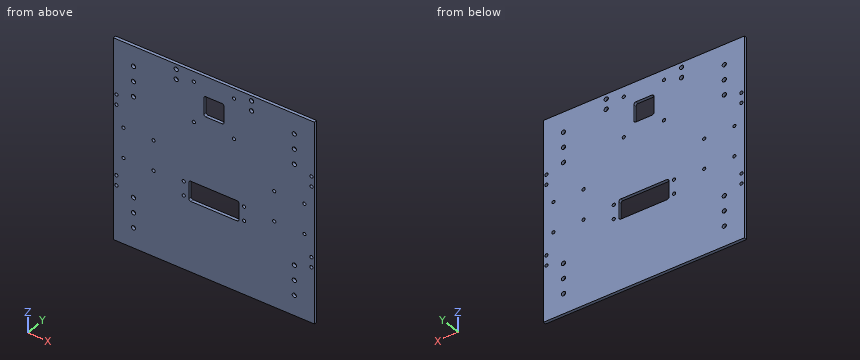
from build123d import *

# Parameters (mm, degrees)
SKETCH_1_W      = 200
SKETCH_1_H      = 200
SKETCH_1_R      = 1.6
SKETCH_1_R_2    = 2.1
EXTRUDE_1_DEPTH = 3


with BuildPart() as part:
    # 草图1 → 凸台-拉伸1 (new body)
    with BuildSketch(Plane(origin=(0, 0, 0), x_dir=(1, 0, 0), z_dir=(0, 1, 0))):
        Rectangle(SKETCH_1_W, SKETCH_1_H)
        with Locations(Location((-97, 35, 0), (0, 0, 270))):
            Circle(SKETCH_1_R, mode=Mode.SUBTRACT)
        with Locations(Location((-97, 45, 0), (0, 0, 270))):
            Circle(SKETCH_1_R, mode=Mode.SUBTRACT)
        with Locations(Location((-97, -45, 0), (0, 0, 90))):
            Circle(SKETCH_1_R, mode=Mode.SUBTRACT)
        with Locations(Location((-97, -35, 0), (0, 0, 90))):
            Circle(SKETCH_1_R, mode=Mode.SUBTRACT)
        with Locations(Location((97, -45, 0), (0, 0, 270))):
            Circle(SKETCH_1_R, mode=Mode.SUBTRACT)
        with Locations(Location((97, -35, 0), (0, 0, 270))):
            Circle(SKETCH_1_R, mode=Mode.SUBTRACT)
        with Locations(Location((97, 35, 0), (0, 0, 90))):
            Circle(SKETCH_1_R, mode=Mode.SUBTRACT)
        with Locations(Location((97, 45, 0), (0, 0, 90))):
            Circle(SKETCH_1_R, mode=Mode.SUBTRACT)
        with Locations(Location((-37.5, -95, 0), (0, 0, 270))):
            Circle(SKETCH_1_R_2, mode=Mode.SUBTRACT)
        with Locations(Location((-37.5, -85, 0), (0, 0, 270))):
            Circle(SKETCH_1_R_2, mode=Mode.SUBTRACT)
        with Locations(Location((37.5, -85, 0), (0, 0, 90))):
            Circle(SKETCH_1_R_2, mode=Mode.SUBTRACT)
        with Locations(Location((37.5, -95, 0), (0, 0, 90))):
            Circle(SKETCH_1_R_2, mode=Mode.SUBTRACT)
        with Locations(Location((-20, -50, 0), (0, 0, 270))):
            Circle(SKETCH_1_R, mode=Mode.SUBTRACT)
        with Locations(Location((20, -50, 0), (0, 0, 270))):
            Circle(SKETCH_1_R, mode=Mode.SUBTRACT)
        with Locations(Location((20, -90, 0), (0, 0, 270))):
            Circle(SKETCH_1_R, mode=Mode.SUBTRACT)
        with Locations(Location((-20, -90, 0), (0, 0, 270))):
            Circle(SKETCH_1_R, mode=Mode.SUBTRACT)
        with Locations(Location((-30, 27, 0), (0, 0, 270))):
            Circle(SKETCH_1_R, mode=Mode.SUBTRACT)
        with Locations(Location((-30, 13, 0), (0, 0, 270))):
            Circle(SKETCH_1_R, mode=Mode.SUBTRACT)
        with Locations(Location((30, 13, 0), (0, 0, 90))):
            Circle(SKETCH_1_R, mode=Mode.SUBTRACT)
        with Locations(Location((30, 27, 0), (0, 0, 90))):
            Circle(SKETCH_1_R, mode=Mode.SUBTRACT)
        with Locations(Location((-80, 50, 0), (0, 0, 270))):
            Circle(SKETCH_1_R_2, mode=Mode.SUBTRACT)
        with Locations(Location((-80, 65, 0), (0, 0, 270))):
            Circle(SKETCH_1_R_2, mode=Mode.SUBTRACT)
        with Locations(Location((-80, 80, 0), (0, 0, 270))):
            Circle(SKETCH_1_R_2, mode=Mode.SUBTRACT)
        with Locations(Location((80, 80, 0), (0, 0, 90))):
            Circle(SKETCH_1_R_2, mode=Mode.SUBTRACT)
        with Locations(Location((80, 65, 0), (0, 0, 90))):
            Circle(SKETCH_1_R_2, mode=Mode.SUBTRACT)
        with Locations(Location((80, 50, 0), (0, 0, 90))):
            Circle(SKETCH_1_R_2, mode=Mode.SUBTRACT)
        with Locations(Location((80, -80, 0), (0, 0, 270))):
            Circle(SKETCH_1_R_2, mode=Mode.SUBTRACT)
        with Locations(Location((80, -65, 0), (0, 0, 270))):
            Circle(SKETCH_1_R_2, mode=Mode.SUBTRACT)
        with Locations(Location((80, -50, 0), (0, 0, 270))):
            Circle(SKETCH_1_R_2, mode=Mode.SUBTRACT)
        with Locations(Location((-80, -80, 0), (0, 0, 90))):
            Circle(SKETCH_1_R_2, mode=Mode.SUBTRACT)
        with Locations(Location((-80, -65, 0), (0, 0, 90))):
            Circle(SKETCH_1_R_2, mode=Mode.SUBTRACT)
        with Locations(Location((-80, -50, 0), (0, 0, 90))):
            Circle(SKETCH_1_R_2, mode=Mode.SUBTRACT)
        with Locations(Location((-90, 15, 0), (0, 0, 270))):
            Circle(SKETCH_1_R, mode=Mode.SUBTRACT)
        with Locations(Location((-60, 15, 0), (0, 0, 270))):
            Circle(SKETCH_1_R, mode=Mode.SUBTRACT)
        with Locations(Location((-60, -15, 0), (0, 0, 270))):
            Circle(SKETCH_1_R, mode=Mode.SUBTRACT)
        with Locations(Location((-90, -15, 0), (0, 0, 270))):
            Circle(SKETCH_1_R, mode=Mode.SUBTRACT)
        with Locations(Location((90, -15, 0), (0, 0, 90))):
            Circle(SKETCH_1_R, mode=Mode.SUBTRACT)
        with Locations(Location((60, -15, 0), (0, 0, 90))):
            Circle(SKETCH_1_R, mode=Mode.SUBTRACT)
        with Locations(Location((60, 15, 0), (0, 0, 90))):
            Circle(SKETCH_1_R, mode=Mode.SUBTRACT)
        with Locations(Location((90, 15, 0), (0, 0, 90))):
            Circle(SKETCH_1_R, mode=Mode.SUBTRACT)
        with BuildLine():
            Line((-23, 10), (23, 10))
            ThreePointArc((23, 10), (24.414213562, 10.585786438), (25, 12))
            Line((25, 12), (25, 28))
            ThreePointArc((25, 28), (24.414213562, 29.414213562), (23, 30))
            Line((23, 30), (-23, 30))
            ThreePointArc((-23, 30), (-24.414213562, 29.414213562), (-25, 28))
            Line((-25, 28), (-25, 12))
            ThreePointArc((-25, 12), (-24.414213562, 10.585786438), (-23, 10))
        make_face(mode=Mode.SUBTRACT)
        with BuildLine():
            Line((-8, -80), (8, -80))
            ThreePointArc((8, -80), (9.414213562, -79.414213562), (10, -78))
            Line((10, -78), (10, -62))
            ThreePointArc((10, -62), (9.414213562, -60.585786438), (8, -60))
            Line((8, -60), (-8, -60))
            ThreePointArc((-8, -60), (-9.414213562, -60.585786438), (-10, -62))
            Line((-10, -62), (-10, -78))
            ThreePointArc((-10, -78), (-9.414213562, -79.414213562), (-8, -80))
        make_face(mode=Mode.SUBTRACT)
    extrude(amount=EXTRUDE_1_DEPTH)


solid = part.part
Here's how the part is built. I have some questions about the finished solid (model axes, mm). Round coordinates to 2 decimals unless told otherwise and drop trailing zeros. Return JSON: item names as keys, results as strings. Group by question number.
1. Please list where these lines run through material, in increasing order: probe 1 along X at (y, z) = (1.9, 35); probe 2 along Z at (x, y) = (97, 1.45); probe 3 along X at (y, z) = (2.3, 90).
2. If we section it at A-A on y = 2.3: State how many separate pieces and enclosed holes the cut face has, then the cut area to 3 significant figures.
3. I'm going to push a flat-ended pin straight in: pin 1 Ø4 at (x, z) = (-31, -78.5) entering from -Y. Where does the tip first touch, or does it pass through?
Reply:
{
 "1": {"probe 1": "-100 to -98.6, -95.4 to 95.4, 98.6 to 100", "probe 2": "-100 to -46.6, -43.4 to -36.6, -33.4 to 33.4, 36.6 to 43.4, 46.6 to 100", "probe 3": "-100 to -21.6, -18.4 to 18.4, 21.6 to 100"},
 "2": {"separate pieces": "1", "enclosed holes": "42", "area": "38,200 mm^2"},
 "3": {"pin 1": "y = 0"}
}
